The listing builds one solid part. Answer for the finished solid, in the listing's coordinates (mm). A direction names the side the tool comes from. Round coordinates to 2 decimals unless told otherwise and drop trailing zeros. Write each loop counter-clockwise with the first axis right and the second up, starting at its lowest first coordinate (ties: lowest second). Pieces come first, ordered by that corner, then holes. Notation, with made-up numbers: (-19, 68.5) - (14, 68.5) arc R10 cw to (14, 73.5) - close; hole circle Ø11 at (14, 73). An arc over 180 degrees is marked (long way). Answer in a Markdown table with one row per item.
from build123d import *

# Parameters (mm, degrees)
PAD_DEPTH          = 9
SKETCH001_W        = 26.1
SKETCH001_H        = 34.4
POCKET_DEPTH       = 3
SKETCH002_R        = 22.22
PAD001_DEPTH       = 3
SKETCH003_R        = 24.44
PAD002_DEPTH       = 3
SKETCH004_R        = 26.6
PAD003_DEPTH       = 3
SKETCH005_R        = 28
PAD004_DEPTH       = 3
SKETCH006_R        = 29
PAD005_DEPTH       = 3
SKETCH007_R        = 29
PAD006_DEPTH       = 3
SKETCH008_R        = 29
PAD007_DEPTH       = 3
SKETCH009_W        = 17
SKETCH009_H        = 24
POCKET001_DEPTH    = 3
SKETCH010_W        = 16
SKETCH010_H        = 9
POCKET002_DEPTH    = 7
SKETCH011_W        = 20
SKETCH011_H        = 9
POCKET003_DEPTH    = 3
SKETCH012_R        = 1.25
POCKET004_DEPTH    = 270.433943
POLARPATTERN_COUNT = 6
SKETCH013_W        = 3
SKETCH013_H        = 38
POCKET005_DEPTH    = 3
SKETCH014_W        = 3
SKETCH014_H        = 6
POCKET006_DEPTH    = 6
SKETCH015_W        = 10.05
SKETCH015_H        = 6
POCKET007_DEPTH    = 3


with BuildPart() as part:
    # Sketch → Pad (new body)
    with BuildSketch(Plane.XY):
        Polygon((44, 0), (22, 38.105118), (-22, 38.105118), (-44, 0), (-22, -38.105118), (22, -38.105118), align=None)
    extrude(amount=PAD_DEPTH)

    # Sketch001 (on Face8 of Pad) → Pocket (cut)
    with BuildSketch(Plane.XY.offset(9)):
        with Locations((0, -13.905118)):
            Rectangle(SKETCH001_W, SKETCH001_H)
    extrude(amount=-POCKET_DEPTH, mode=Mode.SUBTRACT)

    # Sketch002 (on Face5 of Pocket) → Pad001 (join)
    with BuildSketch(Plane.XY.offset(9)):
        Polygon((22, 38.105118), (-22, 38.105118), (-44, 0), (-22, -38.105118), (22, -38.105118), (44, 0), align=None)
        Circle(SKETCH002_R, mode=Mode.SUBTRACT)
    extrude(amount=PAD001_DEPTH)

    # Sketch003 (on Face14 of Pad001) → Pad002 (join)
    with BuildSketch(Plane.XY.offset(12)):
        Polygon((40, 0), (20, 34.641016), (-20, 34.641016), (-40, 0), (-20, -34.641016), (20, -34.641016), align=None)
        Circle(SKETCH003_R, mode=Mode.SUBTRACT)
    extrude(amount=PAD002_DEPTH)

    # Sketch004 (on Face21 of Pad002) → Pad003 (join)
    with BuildSketch(Plane.XY.offset(15)):
        Polygon((41, 0), (20.5, 35.507042), (-20.5, 35.507042), (-41, 0), (-20.5, -35.507042), (20.5, -35.507042), align=None)
        Circle(SKETCH004_R, mode=Mode.SUBTRACT)
    extrude(amount=PAD003_DEPTH)

    # Sketch005 (on Face28 of Pad003) → Pad004 (join)
    with BuildSketch(Plane.XY.offset(18)):
        Polygon((19, 32.908965), (-19, 32.908965), (-38, 0), (-19, -32.908965), (19, -32.908965), (38, 0), align=None)
        Circle(SKETCH005_R, mode=Mode.SUBTRACT)
    extrude(amount=PAD004_DEPTH)

    # Sketch006 (on Face35 of Pad004) → Pad005 (join)
    with BuildSketch(Plane.XY.offset(21)):
        Polygon((39, 0), (19.5, 33.774991), (-19.5, 33.774991), (-39, 0), (-19.5, -33.774991), (19.5, -33.774991), align=None)
        Circle(SKETCH006_R, mode=Mode.SUBTRACT)
    extrude(amount=PAD005_DEPTH)

    # Sketch007 (on Face42 of Pad005) → Pad006 (join)
    with BuildSketch(Plane.XY.offset(24)):
        Polygon((36, 0), (18, 31.176915), (-18, 31.176915), (-36, 0), (-18, -31.176915), (18, -31.176915), align=None)
        Circle(SKETCH007_R, mode=Mode.SUBTRACT)
    extrude(amount=PAD006_DEPTH)

    # Sketch008 (on Face49 of Pad006) → Pad007 (join)
    with BuildSketch(Plane.XY.offset(27)):
        Polygon((37, 0), (18.5, 32.04294), (-18.5, 32.04294), (-37, 0), (-18.5, -32.04294), (18.5, -32.04294), align=None)
        Circle(SKETCH008_R, mode=Mode.SUBTRACT)
    extrude(amount=PAD007_DEPTH)

    # Sketch009 (on Face74 of Pad007) → Pocket001 (cut)
    with BuildSketch(Plane.XY.offset(6)):
        with Locations((0, -8.705118)):
            Rectangle(SKETCH009_W, SKETCH009_H)
    extrude(amount=-POCKET001_DEPTH, mode=Mode.SUBTRACT)

    # Sketch010 (on Face12 of Pocket001) → Pocket002 (cut)
    with BuildSketch(Plane.XZ.offset(38.105118)):
        with Locations((0, 7.5)):
            Rectangle(SKETCH010_W, SKETCH010_H)
    extrude(amount=-POCKET002_DEPTH, mode=Mode.SUBTRACT)

    # Sketch011 (on Face40 of Pocket002) → Pocket003 (cut)
    with BuildSketch(Plane.XY.offset(9)):
        with Locations((0, 17.72)):
            Rectangle(SKETCH011_W, SKETCH011_H)
    extrude(amount=-POCKET003_DEPTH, mode=Mode.SUBTRACT)

    # Sketch012 (on Face93 of Pocket003) → Pocket004 (cut, through all)
    with BuildSketch(Plane.XY.offset(30)):
        with Locations((-32.33, 0)):
            Circle(SKETCH012_R)
    pocket004 = extrude(amount=-POCKET004_DEPTH, mode=Mode.SUBTRACT)

    # PolarPattern: Pocket004 ×6 about axis
    polarpattern_axis = Axis((0, 0, 30), (0, 0, 1))
    for i in range(1, POLARPATTERN_COUNT):
        add(pocket004.rotate(polarpattern_axis, i * 360 / POLARPATTERN_COUNT), mode=Mode.SUBTRACT)

    # Sketch013 (on Face45 of PolarPattern) → Pocket005 (cut)
    with BuildSketch(Plane.XY.offset(6)):
        with Locations((-11.55, -12.105118)):
            Rectangle(SKETCH013_W, SKETCH013_H)
    extrude(amount=-POCKET005_DEPTH, mode=Mode.SUBTRACT)

    # Sketch014 (on Face58 of Pocket005) → Pocket006 (cut)
    with BuildSketch(Plane.XY.offset(9)):
        with Locations((-11.55, 6.294882)):
            Rectangle(SKETCH014_W, SKETCH014_H)
    extrude(amount=-POCKET006_DEPTH, mode=Mode.SUBTRACT)

    # Sketch015 (on Face58 of Pocket006) → Pocket007 (cut)
    with BuildSketch(Plane.XY.offset(9)):
        with Locations((-5.025, 6.294882)):
            Rectangle(SKETCH015_W, SKETCH015_H)
    extrude(amount=-POCKET007_DEPTH, mode=Mode.SUBTRACT)


solid = part.part
(1) Section B-B (z = 2) is taken. Give the vertices of the cut face in (x, y) (3 decimals).
Checked values:
| item | result |
|---|---|
| outline | (-44, 0) - (-22, -38.105) - (22, -38.105) - (44, 0) - (22, 38.105) - (-22, 38.105) - close; hole circle Ø2.5 at (-32.33, 0); hole circle Ø2.5 at (-16.165, -27.999); hole circle Ø2.5 at (-16.165, 27.999); hole circle Ø2.5 at (16.165, -27.999); hole circle Ø2.5 at (16.165, 27.999); hole circle Ø2.5 at (32.33, 0) |
(2) For faces 4 (the flat face through (27.88, 15.8, 28.48)), 5 (the flat face through (-29.386, -16.651, 22.479)), 6 (the flat face through (0, 22.22, 8)), 7 (the cylindrical face through (25.865, -10.724, 19.479)), 8 (the flat face through (0, 33.775, 22)), determine the directions among +Z, -Z, +X, -X, +Y, -Y from which every point of the face is accessible in a straight line to the end or side of a thin tool.
Checked values:
| item | result |
|---|---|
| face 4 | +Z, +X, +Y |
| face 5 | +Z, -X, -Y |
| face 6 | none |
| face 7 | +Z |
| face 8 | +Z, +X, -X, +Y |
(3) Flat-ended cylindrical pins translate along their axes: pin 1 (1.5 mm diameter, centred on x = 2, y = 18, fed in from +Z); pin 2 (0.9 mm diameter, centred on y = -20.5, z = 4.5, fed in from -X); pin 3 (5 mm diameter, centred on y = 14, z = 21, fed in from +X). Find the tip coordinate at first contact, or state that the pin passes through.
Checked values:
| item | result |
|---|---|
| pin 1 | stops at z = 6 |
| pin 2 | stops at x = -32.42 |
| pin 3 | stops at x = 32.36 |
(4) Find the intervals of material crossed by line 1 (Y direction, x = 4, z = 6.75); line 2 (Z direction, x = 34, y = 7); line 3 (Y direction, x = -1, z = 24.75), in increasing order.
Checked values:
| item | result |
|---|---|
| line 1 | y = 3.29 to 13.22, 22.22 to 38.11 |
| line 2 | z = 0 to 18, 21 to 24 |
| line 3 | y = -31.18 to -28.98, 28.98 to 31.18 |
(5) For a pull along X with two mould halves and no side action, classify faces 1 (the flat face through (27.62, -16.25, 28.48)), 2 (the cylindrical face through (13.38, -25.73, 25.44)), 3 (the flat face through (-28.37, 16.68, 19.48)) as pulls with the +X half, pulls with the -X half, needs draft (parallel to the pull), parting line crosses it, or undercut.
Checked values:
| item | result |
|---|---|
| face 1 | pulls with the +X half |
| face 2 | undercut |
| face 3 | pulls with the -X half |
